The model under review builds one solid part; all positions refer to its coordinate system, in mm. A direction names the side the tool comes from. Round coordinates to 2 decimals unless told otherwise and drop trailing zeros. Write each loop counter-clockwise with the first axis right and the second up, starting at its lowest first coordinate (ties: lowest second). Pieces come first, ordered by that corner, then holes. Notation, with made-up numbers: (85, 67.5) -> (140, 67.5) arc R19 ccw to (140, 97.5) -> close; hole circle Ø6 at (18.5, 18.25). An arc over 180 degrees is marked (long way). Answer in a Markdown table with one row per item. Add a question column.
```python
from build123d import *

# Parameters (mm, degrees)
SKETCH1_R           = 2.25
BOSS_EXTRUDE1_DEPTH = 2
FILLET1_R           = 10.25
FILLET2_R           = 2
SKETCH2_R           = 1.5
SKETCH2_W           = 4
SKETCH2_H           = 2
CUT_EXTRUDE1_DEPTH  = 2
FILLET3_R           = 8


with BuildPart() as part:
    # Sketch1 → Boss-Extrude1 (new body)
    with BuildSketch(Plane(origin=(0, 0, 0), x_dir=(1, 0, 0), z_dir=(0, 1, 0))):
        Polygon((0, 0), (37.5, 0), (37.5, -10.25), (65.5, -10.25), (65.5, -0.75), (65.5, 21.25), (65.5, 30.75), (37.5, 30.75), (37.5, 20.5), (0, 20.5), align=None)
        with Locations(Location((10.25, 10.25, 0), (0, 0, 270))):
            Circle(SKETCH1_R, mode=Mode.SUBTRACT)
    extrude(amount=BOSS_EXTRUDE1_DEPTH)

    # Fillet1
    fillet1_edges = [part.edges().sort_by_distance(p)[0] for p in [
        (0, 1, -20.5),
        (0, 1, 0),
    ]]
    fillet(fillet1_edges, radius=FILLET1_R - 0.0001)  # a hair under: the kernel refuses the full size

    # Fillet2
    fillet2_edges = [part.edges().sort_by_distance(p)[0] for p in [
        (37.5, 1, -30.75),
        (65.5, 1, -30.75),
        (65.5, 1, 10.25),
        (37.5, 1, 10.25),
    ]]
    fillet(fillet2_edges, radius=FILLET2_R)

    # Sketch2 → Cut-Extrude1 (cut)
    with BuildSketch(Plane(origin=(0, 2, 0), x_dir=(1, 0, 0), z_dir=(0, 1, 0))):
        with Locations(Location((51.5, 28.75, 0), (0, 0, 270))):
            Circle(SKETCH2_R)
        with Locations(Location((51.5, 10.25, 0), (0, 0, 270))):
            Circle(SKETCH2_R)
        with Locations(Location((51.5, -8.25, 0), (0, 0, 270))):
            Circle(SKETCH2_R)
        with Locations((44.5, 28.75)):
            Rectangle(SKETCH2_W, SKETCH2_H)
        with Locations((58.5, 28.75)):
            Rectangle(SKETCH2_W, SKETCH2_H)
        with Locations((44.5, 10.25)):
            Rectangle(SKETCH2_W, SKETCH2_H)
        with Locations((58.5, 10.25)):
            Rectangle(SKETCH2_W, SKETCH2_H)
        with Locations((44.5, -8.25)):
            Rectangle(SKETCH2_W, SKETCH2_H)
        with Locations((58.5, -8.25)):
            Rectangle(SKETCH2_W, SKETCH2_H)
    extrude(amount=-CUT_EXTRUDE1_DEPTH, mode=Mode.SUBTRACT)

    # Fillet3
    fillet3_edges = [part.edges().sort_by_distance(p)[0] for p in [
        (37.5, 1, -20.5),
        (37.5, 1, 0),
    ]]
    fillet(fillet3_edges, radius=FILLET3_R)


solid = part.part
```
1. Add section A-A on x = 43.5. Write out the cut boundary in (y, z), plus the area to 3 significant figures.
2. Insertion check: pin 1 Ø1 at (y, z) = (1, 8.5) entering from -X; pin 2 Ø3.5 at (x, z) = (51.5, -28.75) entering from -Y. Each pin has a flat end and moves straight along its axis. Give the tip position at first contact, or say it passes through.
3. Add section D-D on z = -25. Write out the cut boundary in (x, y).
4. Add section B-B on y = 0.7. State how many separate pieces and enclosed holes the cut face has, plus the area to 3 significant figures.
5. Mouldability with a two-part tool opening along X and no side actions: class faces 3 (the cylindrical face through (35.094, 1.014, -22.781)), 4 (the flat face through (20, 1, 0)), 5 (the flat face through (44, 1, -9.25)) as pulls with the +X half, pulls with the -X half, needs draft (parallel to the pull), parting line crosses it, or undercut.
6. For L1, parallel to X at y = 1, z = -28.75; L2, parallel to Z at x = 60, y = 0.45; L3, parallel to X at y = 1.2, z = -10.25, list the stretches that pass through material, from the lowest coordinate up.
7. Add section C-C on x = 51.5. Write out the cut boundary in (y, z), plus the area to 3 significant figures.
8. Tool access review of faces 1 (the flat face through (58, 1, -29.75)), 2 (the cylindrical face through (38.1, 1.01, -30.18)): name each direction out of +Z, -Z, +X, -X, +Y, -Y from which nothing blocks a thin tool from reaching the whole face with its end or side.
Filled in:
| question | item | result |
|---|---|---|
| 1 | outline | (0, -30.75) -> (2, -30.75) -> (2, -29.75) -> (0, -29.75) -> close; (0, -27.75) -> (2, -27.75) -> (2, -11.25) -> (0, -11.25) -> close; (0, -9.25) -> (2, -9.25) -> (2, 7.25) -> (0, 7.25) -> close; (0, 9.25) -> (2, 9.25) -> (2, 10.25) -> (0, 10.25) -> close |
| 1 | area | 70.0 mm² |
| 2 | pin 1 | x = 37.5 |
| 2 | pin 2 | y = 0 |
| 3 | outline | (36.69, 0) -> (65.5, 0) -> (65.5, 2) -> (36.69, 2) -> close |
| 4 | separate pieces | 1 |
| 4 | enclosed holes | 10 |
| 4 | area | 1,810 mm² |
| 5 | face 3 | pulls with the -X half |
| 5 | face 4 | needs draft |
| 5 | face 5 | undercut |
| 6 | L1 | 37.5 to 42.5, 46.5 to 50, 53 to 56.5, 60.5 to 65.5 |
| 6 | L2 | -30.75 to -29.75, -27.75 to -11.25, -9.25 to 7.25, 9.25 to 10.25 |
| 6 | L3 | 0 to 8, 12.5 to 42.5, 46.5 to 50, 53 to 56.5, 60.5 to 65.5 |
| 7 | outline | (0, -30.75) -> (2, -30.75) -> (2, -30.25) -> (0, -30.25) -> close; (0, -27.25) -> (2, -27.25) -> (2, -11.75) -> (0, -11.75) -> close; (0, -8.75) -> (2, -8.75) -> (2, 6.75) -> (0, 6.75) -> close; (0, 9.75) -> (2, 9.75) -> (2, 10.25) -> (0, 10.25) -> close |
| 7 | area | 64.0 mm² |
| 8 | face 1 | +Y, -Y |
| 8 | face 2 | -Z, -X, +Y, -Y |
